```python
from build123d import *

# Parameters (mm, degrees)
F0_W      = 62
F0_H      = 95
F1_DEPTH  = 9
F2_SIZE   = 5
F3_T      = -2
F5_DEPTH  = 2
F7_DEPTH  = 2
F8_DEPTH  = 25
F10_DEPTH = 90
F12_DEPTH = 3


with BuildPart() as f1:
    # F0 (on Top) → F1 (new body)
    with BuildSketch(Plane.XY):
        Rectangle(F0_W, F0_H)
    extrude(amount=F1_DEPTH)

    # F2
    f2_edges = [f1.edges().sort_by_distance(p)[0] for p in [
        (-31, -47.5, 4.5),
        (31, -47.5, 4.5),
    ]]
    chamfer(f2_edges, length=F2_SIZE)

    # F3
    f3_openings = [f1.faces().sort_by_distance(p)[0] for p in [
        (0, 0.195368, 9),
    ]]
    offset(amount=F3_T, openings=f3_openings)

    # F4 (on face) → F5 (cut)
    with BuildSketch(Plane.YZ.offset(31)):
        with BuildLine():
            ThreePointArc((27.3, 9), (29.8, 6.5), (32.3, 9))
            Line((32.3, 9), (35.5, 9))
            Line((35.5, 9), (45.5, 5))
            Line((45.5, 5), (47.5, 5))
            Line((47.5, 5), (47.5, 10))
            Line((47.5, 10), (-47.5, 10))
            Line((-47.5, 10), (-47.5, 4))
            Line((-47.5, 4), (-42.5, 4))
            Line((-42.5, 4), (10.5, 9))
            Line((10.5, 9), (17, 9))
            ThreePointArc((17, 9), (19.5, 6.5), (22, 9))
            Line((22, 9), (27.3, 9))
        make_face()
    extrude(amount=-F5_DEPTH, mode=Mode.SUBTRACT)

    # F6 (on face) → F7 (cut)
    with BuildSketch(Plane(origin=(0, 47.5, 0), x_dir=(-1, 0, 0), z_dir=(0, 1, 0))):
        Polygon((-29, 9), (-29, 5), (-25.9392373264, 5), (17.7, 5), (18.9, 3.8), (25, 3.8), (26.2, 5), (31, 5), (31, 9), align=None)
    extrude(amount=-F7_DEPTH, mode=Mode.SUBTRACT)

    # F8 (add): a face of the model
    f8_faces = [f1.faces().sort_by_distance(p)[0] for p in [
        (29, -43.0883975313, 6.5056760177),
    ]]
    extrude(f8_faces, amount=F8_DEPTH)

    # F9 (on face) → F10 (cut)
    with BuildSketch(Plane.YZ.offset(54)):
        Polygon((-42.5, 4), (-41.6715728753, 4.0781535023), (-41.6715728753, 9.3699973077), (-47.5018471479, 9.3699973077), (-47.5018471479, 4), align=None)
    extrude(amount=-F10_DEPTH, mode=Mode.SUBTRACT)

    # F11 (on face) → F12 (cut)
    with BuildSketch(Plane(origin=(-31, 0, 0), x_dir=(0, -1, 0), z_dir=(-1, 0, 0))):
        Polygon((-45.5, 9), (-45.5, 5), (42.5, 4), (42.5568181818, 9), align=None)
    extrude(amount=-F12_DEPTH, mode=Mode.SUBTRACT)


solid = f1.part
```
Geometry: final body of the model. Coordinates: model frame, mm. A direction names the side the tool comes from. Round coordinates to 2 decimals unless told otherwise and drop trailing zeros. Write each loop counter-clockwise with the first axis right and the second up, starting at its lowest first coordinate (ties: lowest second). Pieces come first, ordered by that corner, then holes.
Item 1: Section query C-C (y = 19.5). Return loops of the section in (x, z), plus the area to 3 significant figures.
Item 2: Material intervals for L1, parallel to X at y = 1.5, z = 3.5; L2, parallel to Y at x = 18, z = 3; L3, parallel to Z at x = -12, y = -12.5, sorted ascending.
Item 3: Mould query, pull axis X, two halves, no side actions, for faces 4 (the face through (0, -45.5, 3)), 5 (the face through (0, 47.5, 2)), 6 (the face through (-31, 2, 2)). Classes: +X half, -X half, draft (parallel to the pull), parting line (faces both ways), or undercut.
Item 4: Set-up query: faces 1 (the face through (0, 1, 2)), 2 (the face through (0, -46, 4)), 3 (the face through (-28.5, -45, 2)). Return all of +Z, -Z, +X, -X, +Y, -Y with unobstructed straight access to the full face (end or side cutting, diameter ignored); none if empty.
Item 5: Pin query (flat end, axial travel): P1, Ø1.5, axis at x = -4.5, z = 5, coming from the -Y side; P2, Ø1, axis at x = -29, y = 47, coming from the +Z side; P3, Ø2, axis at x = 0, z = 6.5, coming from the -Y side; P4, Ø8, axis at x = 3, y = -35.5, coming from the +Z side. Return the tip coordinate at first contact, or that it passes through.
Item 6: Section query A-A (z = 7.5). Return loops of the section in (x, y).
Item 7: Section query B-B (x = 18). Return loops of the section in (y, z), plus the area to 3 significant figures.
Completed:
1. outline: (-31, 0) - (31, 0) - (31, 6.5) - (29, 6.5) - (29, 2) - (-29, 2) - (-29, 4.7) - (-31, 4.7) - close
1. area: 138 mm2
2. L1: x = -31 to -29, 29 to 31
2. L2: y = -47.5 to -45.5, 45.5 to 47.5
2. L3: z = 0 to 2
3. face 4: undercut
3. face 5: draft
3. face 6: -X half
4. face 1: +Z
4. face 2: +Z, +X, -X, -Y
4. face 3: +Z, -Z, -X, -Y
5. P1: stops at y = 45.5
5. P2: stops at z = 5
5. P3: passes through
5. P4: stops at z = 2
6. outline: (29, -5.4) - (31, -5.4) - (31, 17.5) - (29, 17.5) - close; (29, 21.5) - (31, 21.5) - (31, 27.8) - (29, 27.8) - close; (29, 31.8) - (31, 31.8) - (31, 39.25) - (29, 39.25) - close
7. outline: (-47.5, 0) - (47.5, 0) - (47.5, 5) - (45.5, 5) - (45.5, 2) - (-45.5, 2) - (-45.5, 4) - (-47.5, 4) - close
7. area: 200 mm2
